Job drawing, mm, ordinate dimensions from the low corner. One solid piece. A direction names the side the tool comes from. Give positions to 0.01 mm unless a question says otherwise; leave off trailing zeros. Loops run counter-clockwise (first coordinate to the right, second up) from the corner with the lowest first, then second, coordinate; pieces in that order, holes last. Notation, with made-up numbers: M 56,0 L 66,0 A20 cw 66,26 Z; hole C 37,79 d11. An arc over 180 degrees is marked long. Answer in a Markdown table with one row per item.
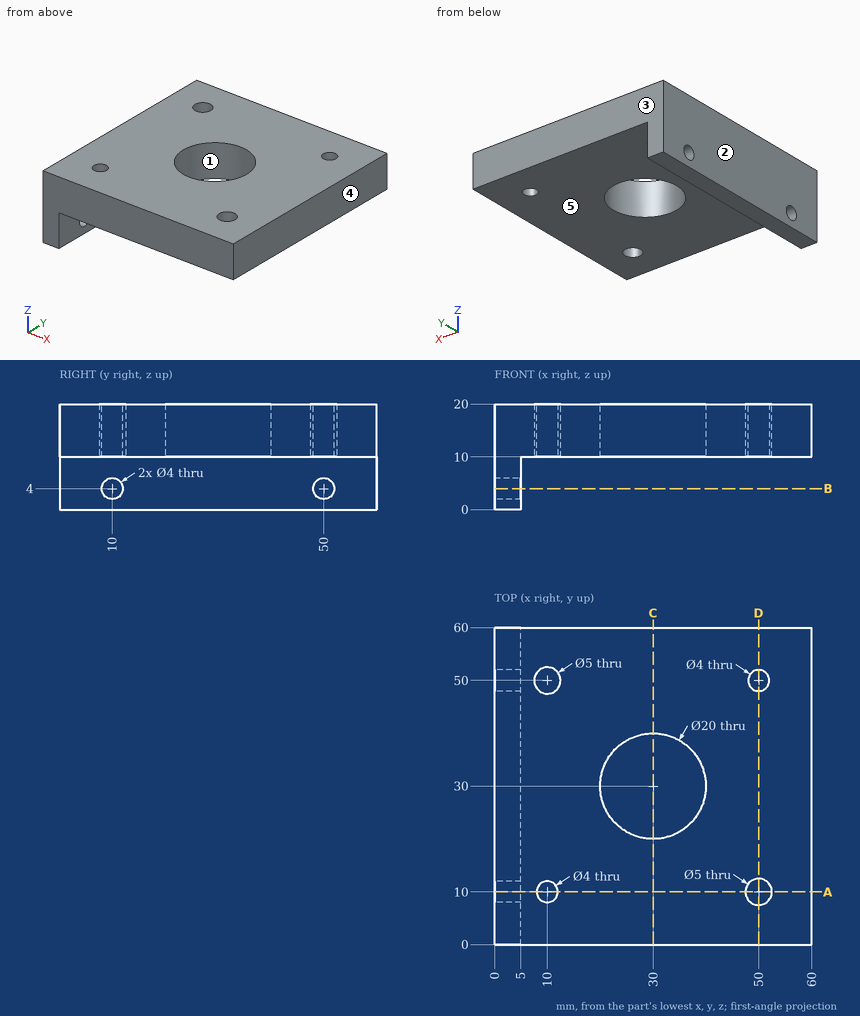
(1) Saw through at C-C (x = 30). Write the cut outline in (y, z), plus the area to 3 significant figures.
Recorded:
| item | result |
|---|---|
| outline | M 0,10 L 20,10 L 20,20 L 0,20 Z; M 40,10 L 60,10 L 60,20 L 40,20 Z |
| area | 400 mm^2 |
(2) Saw through at A-A (y = 10). Write the cut outline in (x, z), plus the area to 3 significant figures.
Recorded:
| item | result |
|---|---|
| outline | M 0,0 L 5,0 L 5,2 L 0,2 Z; M 0,6 L 5,6 L 5,10 L 8,10 L 8,20 L 0,20 Z; M 12,10 L 47.5,10 L 47.5,20 L 12,20 Z; M 52.5,10 L 60,10 L 60,20 L 52.5,20 Z |
| area | 540 mm^2 |
(3) Saw through at B-B (z = 4). Write the cut outline in (x, y).
Recorded:
| item | result |
|---|---|
| outline | M 0,0 L 5,0 L 5,8 L 0,8 Z; M 0,12 L 5,12 L 5,48 L 0,48 Z; M 0,52 L 5,52 L 5,60 L 0,60 Z |
(4) Saw through at D-D (x = 50). Write the cut outline in (y, z), plus the area to 3 significant figures.
Recorded:
| item | result |
|---|---|
| outline | M 0,10 L 7.5,10 L 7.5,20 L 0,20 Z; M 12.5,10 L 48,10 L 48,20 L 12.5,20 Z; M 52,10 L 60,10 L 60,20 L 52,20 Z |
| area | 510 mm^2 |
(5) Pull direction Y, two halves, no side cores. Call the marked faces 1, 2 and 3: +Y half, -Y half, draft (parallel to the pull), parting line (faces both ways), or undercut.
Recorded:
| item | result |
|---|---|
| face 1 | undercut |
| face 2 | draft |
| face 3 | +Y half |
(6) Which spindle directions (+Z, -Z, +X, -X, +Y, -Y) get a long thin tool onto all of the face, cutting with end or side? Do the marked faces 4 and 5. Say none if no direction does.
Recorded:
| item | result |
|---|---|
| face 4 | +Z, -Z, +X, +Y, -Y |
| face 5 | -Z, +X, +Y, -Y |
(7) Drill centre lines: line 1 along Y through (x, z) = (50, 17); line 2 along Y through (x, z) = (1.1, 4); line 3 along Y through (x, z) = (30, 12.5). Where is each one in solid material? Low to high.
Recorded:
| item | result |
|---|---|
| line 1 | y = 0 to 7.5, 12.5 to 48, 52 to 60 |
| line 2 | y = 0 to 8, 12 to 48, 52 to 60 |
| line 3 | y = 0 to 20, 40 to 60 |
(8) Pin check, flat tips, straight feed: pin 1 Ø23 at (x, y) = (30, 30) entering from +Z; pin 2 Ø5 at (y, z) = (29, 7) entering from +X; pin 3 Ø5 at (x, y) = (11.5, 27) entering from -Z; pin 4 Ø3.5 at (y, z) = (10, 4) entering from +X. Stop position of each tip, or through.
Recorded:
| item | result |
|---|---|
| pin 1 | stops at z = 20 |
| pin 2 | stops at x = 5 |
| pin 3 | stops at z = 10 |
| pin 4 | passes through |
